Build history of the part. All positions in model axes, mm. A direction names the side the tool comes from. Coordinates: 2 decimals unless noted, no trailing zeros. Loops run counter-clockwise (first coordinate to the right, second up) from the corner with the lowest first, then second, coordinate; pieces in that order, holes last.
Item 1: 3-axis set-ups, long thin cutter, end or side, ignore diameter. For faces 1 (the face through (26.365, 2, 0)), 2 (the face through (-27, -0.991, 2)), 3 (the face through (30.585, 1.713, -0.225)): which of +Z, -Z, +X, -X, +Y, -Y reach the whole face in a straight line?
Item 2: Mould opens along Z. For faces 4 (the face through (0, 0, -15.875)), 5 (the face through (34.925, 2, 0)), 6 (the face through (-32.54, 1.12, -0.17)) say: released by +Z, released by -Z, zero draft, split by the parting line, or undercut.
Item 3: Cut at B-B (x = 4). List the corners of the cut face in (y, z) (3 decimals).
Item 4: Flat gauge pins, fed straight in: pin 1 (0.9 mm diameter, centred on y = 0, z = 1, fed in from +X); pin 2 (2.5 mm diameter, centred on x = -27, z = 1, fed in from +Y). Where does each tip first touch, or does it go through?
Item 5: Drill centre lines: line 1 along Z through (x, y) = (-18, -1.75) (3 decimals); line 2 along Y through (x, z) = (31.5, 0) (3 decimals); line 3 along Z through (x, y) = (28.5, 0) (3 decimals). Where is each one in solid material? Low to high.
Item 6: Cut at C-C (z = 0). List the corners of the cut face in (x, y) (3 decimals), and give its area (3 significant figures).
from build123d import *

# Parameters (mm, degrees)
SKETCH1_W                                      = 69.85
SKETCH1_H                                      = 31.75
BOSS_EXTRUDE1_DEPTH                            = 3.175
SKETCH2_W                                      = 47.498
SKETCH2_H                                      = 8.128
CUT_EXTRUDE1_DEPTH                             = 6.35
FILLET1_R                                      = 3.175
CBORE_FOR_8_SOCKET_HEAD_CAP_SCREW1_D           = 4.4958
CBORE_FOR_8_SOCKET_HEAD_CAP_SCREW1_DEPTH       = 16.51
CBORE_FOR_8_SOCKET_HEAD_CAP_SCREW1_CBORE_D     = 7.9375
CBORE_FOR_8_SOCKET_HEAD_CAP_SCREW1_CBORE_DEPTH = 4.1656
CBORE_FOR_8_SOCKET_HEAD_CAP_SCREW1_TIP         = 1.350674586
F_8_32_TAPPED_HOLE1_D                          = 3.4544
F_8_32_TAPPED_HOLE1_DEPTH                      = 8.5598


with BuildPart() as part:
    # Sketch1 → Boss-Extrude1 (new, symmetric)
    with BuildSketch(Plane(origin=(0, 0, 0), x_dir=(1, 0, 0), z_dir=(0, 1, 0))):
        Rectangle(SKETCH1_W, SKETCH1_H)
    extrude(amount=BOSS_EXTRUDE1_DEPTH, both=True)

    # Sketch2 → Cut-Extrude1 (cut)
    with BuildSketch(Plane(origin=(0, 3.175, 0), x_dir=(1, 0, 0), z_dir=(0, 1, 0))):
        with Locations((2.6162, 0)):
            Rectangle(SKETCH2_W, SKETCH2_H)
    extrude(amount=-CUT_EXTRUDE1_DEPTH, mode=Mode.SUBTRACT)

    # Fillet1
    fillet1_edges = [part.edges().sort_by_distance(p)[0] for p in [
        (-21.1328, 0, 4.064),
        (-21.1328, 0, -4.064),
        (26.3652, 0, -4.064),
        (26.3652, 0, 4.064),
    ]]
    fillet(fillet1_edges, radius=FILLET1_R)

    # CBORE for #8 Socket Head Cap Screw1
    with Locations(Plane(origin=(0, 3.175, 0), x_dir=(1, 0, 0), z_dir=(0, 1, 0))):
        with Locations((-28.575, 0)):
            CounterBoreHole(CBORE_FOR_8_SOCKET_HEAD_CAP_SCREW1_D / 2, CBORE_FOR_8_SOCKET_HEAD_CAP_SCREW1_CBORE_D / 2, CBORE_FOR_8_SOCKET_HEAD_CAP_SCREW1_CBORE_DEPTH, depth=CBORE_FOR_8_SOCKET_HEAD_CAP_SCREW1_DEPTH)
            with Locations((0, 0, -(CBORE_FOR_8_SOCKET_HEAD_CAP_SCREW1_DEPTH + CBORE_FOR_8_SOCKET_HEAD_CAP_SCREW1_TIP / 2))):  # 118° drill point
                Cone(0, CBORE_FOR_8_SOCKET_HEAD_CAP_SCREW1_D / 2, CBORE_FOR_8_SOCKET_HEAD_CAP_SCREW1_TIP, mode=Mode.SUBTRACT)

    # #8-32 Tapped Hole1
    with Locations(Plane(origin=(34.925, 0, 0), x_dir=(0, 0, -1), z_dir=(1, 0, 0))):
        with Locations((0, 0)):
            Hole(F_8_32_TAPPED_HOLE1_D / 2, depth=F_8_32_TAPPED_HOLE1_DEPTH)


solid = part.part
Filled sheet:
1. face 1: +Y, -Y
1. face 2: +Y
1. face 3: +X
2. face 4: released by -Z
2. face 5: zero draft
2. face 6: undercut
3. outline: (-3.175, -15.875) - (3.175, -15.875) - (3.175, -4.064) - (-3.175, -4.064) - close; (-3.175, 4.064) - (3.175, 4.064) - (3.175, 15.875) - (-3.175, 15.875) - close
4. pin 1: stops at x = 26.37
4. pin 2: stops at y = -0.99
5. line 1: z = -15.875 to -4.064, 4.064 to 15.875
5. line 2: y = -3.175 to -1.727, 1.727 to 3.175
5. line 3: z = -15.875 to -1.727, 1.727 to 15.875
6. outline: (-34.925, -3.175) - (-30.823, -3.175) - (-30.823, -0.991) - (-32.544, -0.991) - (-32.544, 3.175) - (-34.925, 3.175) - close; (-26.327, -3.175) - (-21.133, -3.175) - (-21.133, 3.175) - (-24.606, 3.175) - (-24.606, -0.991) - (-26.327, -0.991) - close; (26.365, -3.175) - (34.925, -3.175) - (34.925, -1.727) - (26.365, -1.727) - close; (26.365, 1.727) - (34.925, 1.727) - (34.925, 3.175) - (26.365, 3.175) - close
6. area: 69.5 mm2
